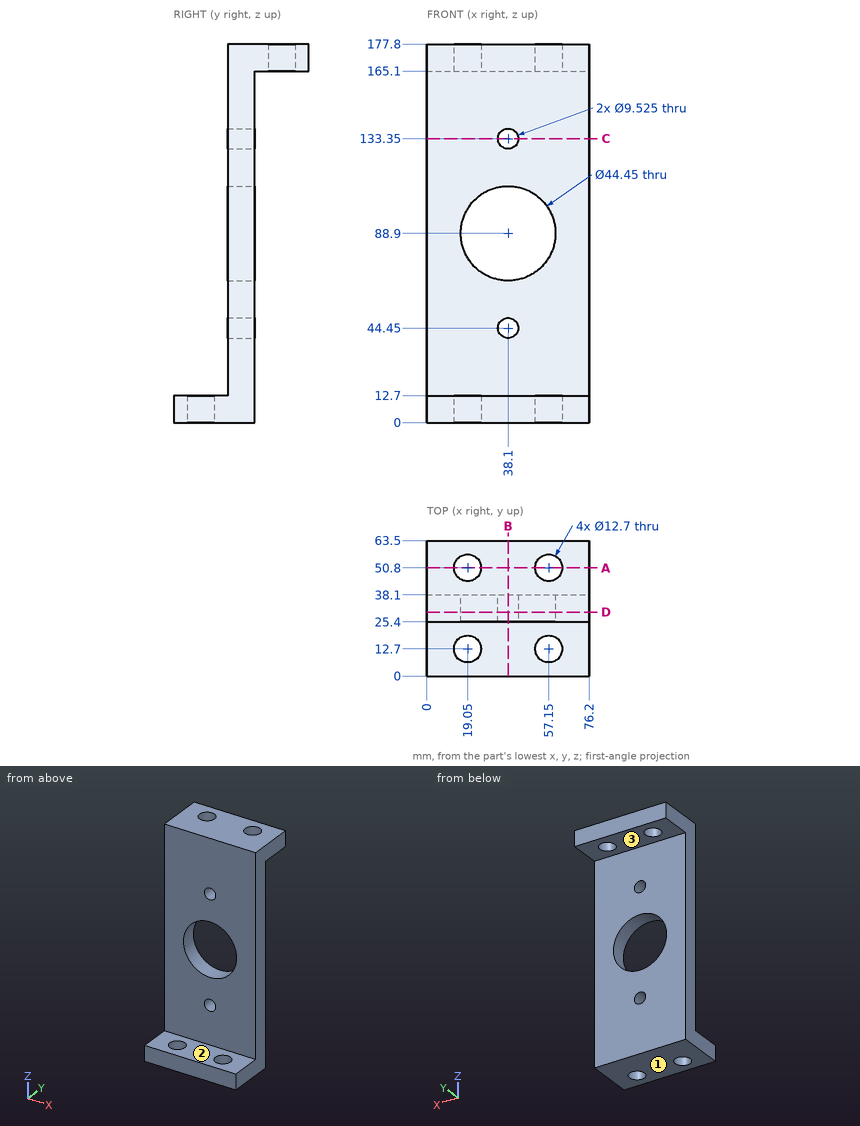
Job drawing, mm, ordinate dimensions from the low corner. One solid piece. A direction names the side the tool comes from. Round coordinates to 2 decimals unless told otherwise and drop trailing zeros. Write each loop counter-clockwise with the first axis right and the second up, starting at its lowest first coordinate (ties: lowest second). Pieces come first, ordered by that corner, then holes. Notation, with made-up numbers: (74, -2.5) -> (132, -2.5) arc R26 ccw to (132, 15.5) -> close; hole circle Ø4 at (38, 57.25). An arc over 180 degrees is marked (long way). Answer as a JSON object with one key per item and string values.
(1) Which spindle directions (+Z, -Z, +X, -X, +Y, -Y) get a long thin tool onto all of the face, cutting with end or side? Do the marked faces 1, 2 and 3. Say none if no direction does.
Reported:
{"face 1": "-Z, +X, -X, +Y, -Y", "face 2": "+Z, +X, -X, -Y", "face 3": "-Z, +X, -X, +Y"}
(2) Band-saw the part on C-C, the plane z = 133.35. List the corners of the cut face in (x, y).
Reported:
{"outline": "(0, 25.4) -> (33.34, 25.4) -> (33.34, 38.1) -> (0, 38.1) -> close; (42.86, 25.4) -> (76.2, 25.4) -> (76.2, 38.1) -> (42.86, 38.1) -> close"}
(3) Probe probe 1 along Z at (x, y) = (38.1, 30) (1 decimal); probe 2 along Y at (x, z) = (19.05, 10.25); probe 3 along Y at (x, z) = (57, 175). List the from-to ranges inside material, lowest first. Write a range as [from, to].
Reported:
{"probe 1": "z = [0, 39.7], [49.2, 66.7], [111.1, 128.6], [138.1, 177.8]", "probe 2": "y = [0, 6.35], [19.05, 38.1]", "probe 3": "y = [25.4, 44.45], [57.15, 63.5]"}
(4) Band-saw the part on B-B, the plane x = 38.1. List the corners of the cut face in (y, z) (1 decimal), then the cut area to 3 significant figures.
Reported:
{"outline": "(0, 0) -> (38.1, 0) -> (38.1, 39.7) -> (25.4, 39.7) -> (25.4, 12.7) -> (0, 12.7) -> close; (25.4, 49.2) -> (38.1, 49.2) -> (38.1, 66.7) -> (25.4, 66.7) -> close; (25.4, 111.1) -> (38.1, 111.1) -> (38.1, 128.6) -> (25.4, 128.6) -> close; (25.4, 138.1) -> (38.1, 138.1) -> (38.1, 165.1) -> (63.5, 165.1) -> (63.5, 177.8) -> (25.4, 177.8) -> close", "area": "2,100 mm^2"}
(5) Band-saw the part on A-A, the plane y = 50.8. List the corners of the cut face in (x, z), then the cut area to 3 significant figures.
Reported:
{"outline": "(0, 165.1) -> (12.7, 165.1) -> (12.7, 177.8) -> (0, 177.8) -> close; (25.4, 165.1) -> (50.8, 165.1) -> (50.8, 177.8) -> (25.4, 177.8) -> close; (63.5, 165.1) -> (76.2, 165.1) -> (76.2, 177.8) -> (63.5, 177.8) -> close", "area": "645 mm^2"}
(6) Band-saw the part on D-D, the plane y = 30. Count the separate pieces of the cut face and the enclosed holes in it, then the cut area to 3 significant figures.
Reported:
{"separate pieces": "1", "enclosed holes": "3", "area": "11,900 mm^2"}
(7) Pin check, flat tips, straight feed: P1, Ø1, axis at y = 23.5, z = 93.5, coming from the +X side; P2, Ø11, axis at x = 38.1, z = 133.35, coming from the +Y side; P3, Ø16.5, axis at x = 19.05, y = 12.7, coming from the -Z side; P4, Ø12.5, axis at x = 38.1, z = 44.45, coming from the -Y side. Stop position of each tip, or through.
Reported:
{"P1": "passes through", "P2": "stops at y = 38.1", "P3": "stops at z = 0", "P4": "stops at y = 25.4"}
